```python
from build123d import *

# Parameters (mm, degrees)
EXTRUDE_8_DEPTH          = 3
EXTRUDE_8_DEPTH_BACK     = 3
SKETCH_3_R               = 2.708293856
EXTRUDE_8_2_DEPTH        = 3
EXTRUDE_8_2_DEPTH_BACK   = 3
CUT_EXTRUDE_1_DEPTH      = 3
CUT_EXTRUDE_1_DEPTH_BACK = 6
SKETCH_4_R               = 1.55
SKETCH_4_R_2             = 1.553894019
SKETCH_7_R               = 1.55
SKETCH_7_R_2             = 1.553894019
EXTRUDE_9_DEPTH          = 1
EXTRUDE_START            = 1
SKETCH_18_R              = 1.55
SKETCH_18_R_2            = 1.553894019
EXTRUDE_17_DEPTH         = 1


with BuildPart() as part:
    # Sketch 3 → Extrude 8 (new, two sides: drawn at the far end of the back side and taken through both)
    with BuildSketch(Plane(origin=(0, 0, 0), x_dir=(1, 0, 0), z_dir=(0, 1, 0)).offset(-EXTRUDE_8_DEPTH_BACK)):
        with Locations(Location((-56.235722287, 24.732868077, 0), (0, 0, 270))):
            Circle(SKETCH_3_R)
    extrude(amount=EXTRUDE_8_DEPTH + EXTRUDE_8_DEPTH_BACK)


with BuildPart() as body_2:
    # Sketch 3 → Extrude 8 2 (new, two sides: drawn at the far end of the back side and taken through both)
    with BuildSketch(Plane(origin=(0, 0, 0), x_dir=(1, 0, 0), z_dir=(0, 1, 0)).offset(-EXTRUDE_8_2_DEPTH_BACK)):
        with Locations(Location((-43.855722287, 24.505707547, 0), (0, 0, 270))):
            Circle(SKETCH_3_R)
    extrude(amount=EXTRUDE_8_2_DEPTH + EXTRUDE_8_2_DEPTH_BACK)


with BuildPart() as cut_extrude_1_tool:
    # Sketch 4 → Cut-Extrude 1 (new, two sides: drawn at the far end of the back side and taken through both)
    with BuildSketch(Plane(origin=(0, 0, 0), x_dir=(1, 0, 0), z_dir=(0, 1, 0)).offset(-CUT_EXTRUDE_1_DEPTH_BACK)):
        with Locations(Location((-56.235722287, 24.732868077, 0), (0, 0, 270))):
            Circle(SKETCH_4_R)
        with Locations(Location((-43.855722287, 24.505707547, 0), (0, 0, 270))):
            Circle(SKETCH_4_R_2)
    extrude(amount=CUT_EXTRUDE_1_DEPTH + CUT_EXTRUDE_1_DEPTH_BACK)


with BuildPart() as part_1:
    add(part.part)

    # Cut-Extrude 1: cut by cut_extrude_1_tool
    add(cut_extrude_1_tool.part, mode=Mode.SUBTRACT)



with BuildPart() as body_2_1:
    add(body_2.part)

    # Cut-Extrude 1: cut by cut_extrude_1_tool
    add(cut_extrude_1_tool.part, mode=Mode.SUBTRACT)


with BuildPart() as part_2:
    add(part_1.part)

    add(body_2_1.part)  # Extrude 9 merges body 2
    # Sketch 7 → Extrude 9 (add)
    # profile 1 of 2: a face of its own
    with BuildSketch(Plane.XZ.offset(3)):
        with BuildLine():
            ThreePointArc((-56.235722287, -20.932868077), (-60.035052689, -24.804201821), (-56.093079937, -28.530189917))
            ThreePointArc((-56.093079937, -28.530189917), (-53.498749422, -27.368959792), (-52.435722287, -24.732868077))
            ThreePointArc((-52.435722287, -24.732868077), (-53.548716519, -22.045862308), (-56.235722287, -20.932868077))
        make_face()
        with Locations(Location((-56.235722287, -24.732868077, 0), (0, 0, 270))):
            Circle(SKETCH_7_R, mode=Mode.SUBTRACT)
    # profile 2 of 2: a face of its own
    with BuildSketch(Plane.XZ.offset(3)):
        with BuildLine():
            ThreePointArc((-43.723017894, -28.303389675), (-41.122201052, -27.145378295), (-40.055722287, -24.505707547))
            ThreePointArc((-40.055722287, -24.505707547), (-41.168716519, -21.818701779), (-43.855722287, -20.705707547))
            add(Edge.make_bspline(
                [(-56.235722287, -20.932868077), (-54.105831048, -20.932868077), (-49.896032342, -22.477788173), (-46.252423284, -20.705707547), (-43.855722287, -20.705707547)],
                knots=[0, 0, 0, 0, 0.498510271, 1, 1, 1, 1], degree=3))
            ThreePointArc((-56.235722287, -20.932868077), (-53.548716519, -22.045862308), (-52.435722287, -24.732868077))
            ThreePointArc((-52.435722287, -24.732868077), (-53.498749422, -27.368959792), (-56.093079937, -28.530189917))
            add(Edge.make_bspline(
                [(-56.093079937, -28.530189917), (-53.942583983, -28.449408827), (-49.768599584, -26.149491118), (-46.433977381, -28.398120151), (-43.723017894, -28.303389675)],
                knots=[0, 0, 0, 0, 0.490575379, 1, 1, 1, 1], degree=3))
        make_face()
        with Locations(Location((-43.855722287, -24.505707547, 0), (0, 0, 90))):
            Circle(SKETCH_7_R_2, mode=Mode.SUBTRACT)
    extrude(amount=EXTRUDE_9_DEPTH)

    # Sketch 18 → Extrude 17 (add)
    with BuildSketch(Plane(origin=(0, 3, 0), x_dir=(1, 0, 0), z_dir=(0, 1, 0)).offset(EXTRUDE_START)):
        with BuildLine():
            ThreePointArc((-56.093079937, 28.530189917), (-60.035052689, 24.804201821), (-56.235722287, 20.932868077))
            add(Edge.make_bspline(
                [(-56.235722287, 20.932868077), (-54.105831048, 20.932868077), (-49.896032342, 22.477788173), (-46.252423284, 20.705707547), (-43.855722287, 20.705707547)],
                knots=[0, 0, 0, 0, 0.498510271, 1, 1, 1, 1], degree=3))
            ThreePointArc((-43.855722287, 20.705707547), (-40.0563018, 24.43934523), (-43.723017894, 28.303389675))
            add(Edge.make_bspline(
                [(-43.723017894, 28.303389675), (-46.433977381, 28.398120151), (-49.768599584, 26.149491118), (-53.942583983, 28.449408827), (-56.093079937, 28.530189917)],
                knots=[0, 0, 0, 0, 0.509424621, 1, 1, 1, 1], degree=3))
        make_face()
        with Locations(Location((-56.235722287, 24.732868077, 0), (0, 0, 90))):
            Circle(SKETCH_18_R, mode=Mode.SUBTRACT)
        with Locations(Location((-43.855722287, 24.505707547, 0), (0, 0, 270))):
            Circle(SKETCH_18_R_2, mode=Mode.SUBTRACT)
    extrude(amount=-EXTRUDE_17_DEPTH)


solid = part_2.part
```
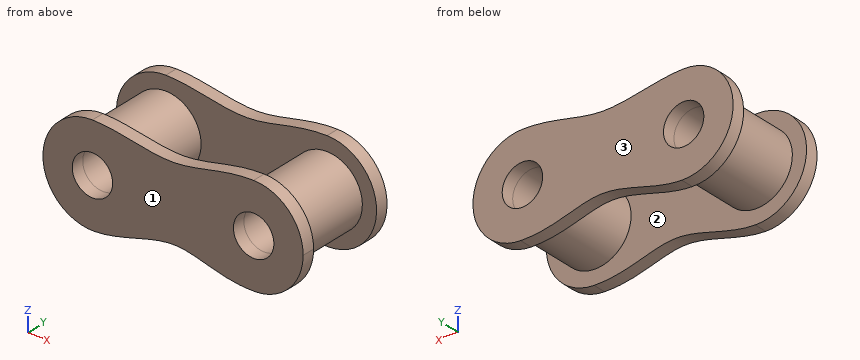
Can you work these out from the model? Positions are in its coordinate system, mm. Face numbers are marked on the shaded views. Coordinates: 2 decimals unless noted, no trailing zeros. Loops run counter-clockwise (first coordinate to the right, second up) from the corner with the lowest first, then second, coordinate; pieces in that order, holes last.
1) Thinking about a two-plate mould opening in Y: for the marked faces 1, 2 and 3, which applies, pulls with the +Y half, pulls with the -Y half, needs draft (parallel to the pull), parting line crosses it, or undercut?
2) Imagine slicing it at A-A on y = 2.5. List the corners of the cut face in (x, z) for me, plus the area to 3 significant figures.
3) Imagine slicing it at C-C on z = -26.75. List the corners of the cut face in (x, y) for me.
4) I need wall thicknesses on probe 1 along X at (y, z) = (2, -24.5); probe 2 along Y at (x, z) = (-43, -27.5); probe 3 along X at (y, z) = (0.75, -23.5). Which ranges of each line are inside material? Lowest first, please.
5) Imagine slicing it at B-B on x = -43.25. List the corners of the cut face in (y, z) for me, plus the area to 3 significant figures.
6) For pin 1 (4 mm diameter, centred on x = -54.5, y = -2.5, fed in from -Z); pin 2 (3 mm diameter, centred on x = -56.24, z = -24.73, fed in from +Y); pin 3 (1 mm diameter, centred on y = 3, z = -27.5, fed in from -X), each with a flat end and sliding along its axis, tell me the tip position at first contact or that it passes through.
Completed:
1. face 1: pulls with the -Y half
1. face 2: undercut
1. face 3: pulls with the +Y half
2. outline: circle Ø5.42 at (-56.24, -24.73); circle Ø5.42 at (-43.86, -24.51); hole circle Ø3.1 at (-56.24, -24.73); hole circle Ø3.11 at (-43.86, -24.51)
2. area: 31.0 mm2
3. outline: (-59.46, -4) - (-40.79, -4) - (-40.79, -3) - (-42.34, -3) - (-42.34, 3) - (-40.79, 3) - (-40.79, 4) - (-59.46, 4) - (-59.46, 3) - (-58.04, 3) - (-58.04, -3) - (-59.46, -3) - close; hole (-54.43, -3) - (-45.37, -3) - (-45.37, 3) - (-54.43, 3) - close
4. probe 1: x = -58.93 to -57.77, -54.7 to -53.54, -46.56 to -45.41, -42.3 to -41.15
4. probe 2: y = -4 to -3, 3 to 4
4. probe 3: x = -58.65 to -57.18, -55.3 to -53.82, -46.37 to -45.04, -42.67 to -41.34
5. outline: (-4, -28.26) - (-3, -28.26) - (-3, -27.15) - (3, -27.15) - (3, -28.26) - (4, -28.26) - (4, -25.94) - (-4, -25.94) - close; (-4, -23.07) - (4, -23.07) - (4, -20.75) - (3, -20.75) - (3, -21.87) - (-3, -21.87) - (-3, -20.75) - (-4, -20.75) - close
5. area: 23.8 mm2
6. pin 1: stops at z = -28.53
6. pin 2: passes through
6. pin 3: stops at x = -59.29
